from build123d import *

# Parameters (mm, degrees)
F0_W     = 508
F0_H     = 285.75
F0_R     = 4.233333
F1_DEPTH = 6.35
F0_H_2   = 6.35
F2_DEPTH = 50.8
F3_W     = 330.2
F3_H     = 165.1
F4_DEPTH = 152.4
F6_DEPTH = 419.101


with BuildPart() as f1:
    # F0 (on Front) → F1 (new body)
    with BuildSketch(Plane.XZ):
        with Locations((-0.770811, -23.840043)):
            Rectangle(F0_W, F0_H)
        with Locations((-223.020811, 106.334957)):
            Circle(F0_R, mode=Mode.SUBTRACT)
        with Locations((-191.270811, 106.334957)):
            Circle(F0_R, mode=Mode.SUBTRACT)
        with Locations((-159.520811, 106.334957)):
            Circle(F0_R, mode=Mode.SUBTRACT)
        with Locations((-127.770811, 106.334957)):
            Circle(F0_R, mode=Mode.SUBTRACT)
        with Locations((-96.020811, 106.334957)):
            Circle(F0_R, mode=Mode.SUBTRACT)
        with Locations((90.245856, 106.334957)):
            Circle(F0_R, mode=Mode.SUBTRACT)
        with Locations((121.995856, 106.334957)):
            Circle(F0_R, mode=Mode.SUBTRACT)
        with Locations((153.745856, 106.334957)):
            Circle(F0_R, mode=Mode.SUBTRACT)
        with Locations((185.495856, 106.334957)):
            Circle(F0_R, mode=Mode.SUBTRACT)
        with Locations((217.245856, 106.334957)):
            Circle(F0_R, mode=Mode.SUBTRACT)
    extrude(amount=F1_DEPTH)

    # F0 (on Front) → F2 (join)
    with BuildSketch(Plane.XZ):
        with Locations((-0.770811, -169.890043)):
            Rectangle(F0_W, F0_H_2)
    extrude(amount=F2_DEPTH)

    # F3 (on face) → F4 (join)
    with BuildSketch(Plane.XZ):
        with Locations((-0.770811, -90.515043)):
            Rectangle(F3_W, F3_H)
    extrude(amount=-F4_DEPTH)

    # F5 (on face) → F6 (cut, through all)
    with BuildSketch(Plane.YZ.offset(164.329189)):
        Polygon((124.205639, -112.185949), (120.123938, -117.050331), (0, -173.065043), (152.4, -173.065043), (152.4, -7.965043), (0, -7.965043), align=None)
        Polygon((120.123938, -117.050331), (0, -16.254379), (0, -173.065043), align=None)
    extrude(amount=-F6_DEPTH, mode=Mode.SUBTRACT)


solid = f1.part
Source: CAD feature listing. Evaluate the final solid. Frame: model axes, mm. A direction names the side the tool comes from. Give positions to 0.01 mm unless a question says otherwise; leave off trailing zeros. Write each loop counter-clockwise with the first axis right and the second up, starting at its lowest first coordinate (ties: lowest second). Pieces come first, ordered by that corner, then holes. Notation, with made-up numbers: (-14.5, 9) - (29.5, 9) arc R14 ccw to (29.5, 20) - close; hole circle Ø4 at (61.5, 80). An arc over 180 degrees is marked (long way). Write item = value, one per line. Start each with the question number.
Q1. Cut plane B-B, the plane z = -105. Return loops of the section in (x, y), then the cut area to 3 significant figures.
Q2. Material intervals for probe 1 along Y at (x, z) = (171.5, -161); probe 2 along Z at (x, y) = (167, -41); probe 3 along Z at (x, y) = (73.5, 114), sorted ascending.
Q3. Pin query (flat end, axial travel): pin 1 Ø2 at (x, z) = (175, 13.5) entering from -Y; pin 2 Ø5 at (x, z) = (102, 88) entering from +Y; pin 3 Ø6 at (y, z) = (-8, -106) entering from +X. Return the tip coordinate at first contact, or that it passes through.
Q4. Cut plane C-C, the plane z = 36. Return loops of the section in (x, y).
Q5. Cut plane D-D, the plane y = -34.5. Return loops of the section in (x, z), then the cut area to 3 significant figures.
Q6. Reachability of faces 1 (the flat face through (164.329, 62, -63)), 2 (the flat face through (-4, -25, -173.065)), 3 (the flat face through (253.229, -5, -60)), 4 (the flat face through (-4, -28, -166.715)), 5 (the flat face through (-165.871, 62, -63)) from +Z, -Z, +X, -X, +Y, -Y: full face, straight path, thin tool, end or side. Return the list, or none.
Q7. Cut plane A-A, the plane x = -66. Return loops of the section in (y, z).
Q8. Draft query along Y for faces 6 (the flat face through (1.541, 61.233, -59.346)), 7 (the flat face through (1.541, 60.903, -67.358)), 8 (the flat face through (-4, -6.35, -22)), 9 (the flat face through (-4, 0, -25)). Return one class per face: +Y half, -Y half, draft (parallel to the pull), parting line (faces both ways), or undercut.
Computed values:
q1.outline = (-254.77, -6.35) - (253.23, -6.35) - (253.23, 0) - (-254.77, 0) - close; (-165.87, 105.76) - (164.33, 105.76) - (164.33, 115.64) - (-165.87, 115.64) - close
q1.area = 6,490 mm²
q2.probe_1 = -6.35 to 0
q2.probe_2 = -173.07 to -166.72
q2.probe_3 = -111.91 to -103.62
q3.pin_1 = -6.35
q3.pin_2 = 0
q3.pin_3 = 253.23
q4.outline = (-254.77, -6.35) - (253.23, -6.35) - (253.23, 0) - (-254.77, 0) - close
q5.outline = (-254.77, -173.07) - (253.23, -173.07) - (253.23, -166.72) - (-254.77, -166.72) - close
q5.area = 3,230 mm²
q6.face_1 = +Z, -Z, +X, +Y
q6.face_2 = -Z, +X, -X, +Y, -Y
q6.face_3 = +Z, -Z, +X, +Y, -Y
q6.face_4 = +Z, +X, -X, -Y
q6.face_5 = +Z, -Z, -X, +Y
q7.outline = (-50.8, -173.07) - (0, -173.07) - (0, -16.25) - (120.12, -117.05) - (124.21, -112.19) - (0, -7.97) - (0, 119.03) - (-6.35, 119.03) - (-6.35, -166.72) - (-50.8, -166.72) - close
q8.face_6 = +Y half
q8.face_7 = undercut
q8.face_8 = -Y half
q8.face_9 = undercut
